```python
from build123d import *

# Parameters (mm, degrees)
SKETCH1_W           = 20
SKETCH1_H           = 40
BOSS_EXTRUDE1_DEPTH = 2


with BuildPart() as part:
    # Sketch1 → Boss-Extrude1 (new body)
    with BuildSketch(Plane.XY):
        Polygon((-50, 20), (-10, 20), (10, 20), (50, 20), (50, 40), (-50, 40), align=None)
        Rectangle(SKETCH1_W, SKETCH1_H)
    extrude(amount=BOSS_EXTRUDE1_DEPTH)


solid = part.part
```
The listing builds one solid part. Answer for the finished solid, in the listing's coordinates (mm). A direction names the side the tool comes from. Give positions to 0.01 mm unless a question says otherwise; leave off trailing zeros. Order: outer loops, then holes, each group sorted by start corner. A loop starts at its lowest first (then second) coordinate and runs counter-clockwise, first axis right, second up.
1) Find section C-C on y = 5.5. Write down the section's boundary in (x, z).
Reported:
outline: (-10, 0) - (10, 0) - (10, 2) - (-10, 2) - close
2) Find section B-B on x = -36. Write down the section's boundary in (y, z), then the cut area to 3 significant figures.
Reported:
outline: (20, 0) - (40, 0) - (40, 2) - (20, 2) - close
area: 40.0 mm2
3) Find section A-A on z = 1.65. Write down the section's boundary in (x, y), then the cut area to 3 significant figures.
Reported:
outline: (-50, 20) - (-10, 20) - (-10, -20) - (10, -20) - (10, 20) - (50, 20) - (50, 40) - (-50, 40) - close
area: 2,800 mm2
4) Given P1, Ø12, axis at x = 12.5, y = 13, coming from the +Z side; P2, Ø1, axis at y = -6, z = 1.5, coming from the -X side; P3, Ø0.6, axis at x = -38.5, z = 1, coming from the -Y side, each flat-ended and moving along its own axis, determine where each tip first touches the part or whether it passes through.
Reported:
P1: stops at z = 2
P2: stops at x = -10
P3: stops at y = 20
5) Consider line 1 along Y through (x, z) = (40, 1.5); line 2 along X through (y, z) = (17.5, 1.45). Determine where each line is inside the solid, lowest interval first.
Reported:
line 1: y = 20 to 40
line 2: x = -10 to 10
6) For faces 1 (the face through (-30, 20, 1)), 2 (the face through (30, 20, 1)), 3 (the face through (1, 40, 1)), determine the directions among +Z, -Z, +X, -X, +Y, -Y from which every point of the face is accessible in a straight line to the end or side of a thin tool.
Reported:
face 1: +Z, -Z, -X, -Y
face 2: +Z, -Z, +X, -Y
face 3: +Z, -Z, +X, -X, +Y
